The drawing under review shows one solid part. Ordinate dimensions are in mm from its lowest x, y, z. A direction names the side the tool comes from. Coordinates: 2 decimals unless noted, no trailing zeros. Write each loop counter-clockwise with the first axis right and the second up, starting at its lowest first coordinate (ties: lowest second). Pieces come first, ordered by that corner, then holes. Notation, with made-up numbers: (8.25, -16.75) -> (62.25, -16.75) arc R17 ccw to (62.25, -4.75) -> close; hole circle Ø10 at (76, 34). An arc over 180 degrees is marked (long way). One line per item, written item: value. Start each with the question number.
1) Add section D-D (y = 9). State the section outline as (x, z) points, and give its area (3 significant figures).
2) Mouldability with a two-part tool opening along X and no side actions: class the marked faces 1, 2 and 3 as released by +X, released by -X, zero draft, split by the parting line, or undercut.
3) For probe 1 along Y at (x, z) = (23, 1.9); probe 2 along X at (y, z) = (4, 13.5); probe 3 along Z at (x, y) = (23, 12.5), list the stretches that pass through material, from the lowest coordinate up. Write a range as from..to.
4) Add section A-A (z = 6.75). State the section outline as (x, y) points.
5) Add section B-B (x = 15). State the section outline as (y, z) points, and give its area (3 significant figures).
6) Add section C-C (y = 3). State the section outline as (x, z) points, and give its area (3 significant figures).
7) For pin 1 Ø2 at (x, y) = (30.5, 20) entering from +Z, flat-tipped, find the tip position at first contact; note if it passes through.
8) Machinability: for the marked faces 4 and 5, which of the approach directions +Z, -Z, +X, -X, +Y, -Y give a long, thin tool a straight path to every point of the face, cutting with its end or side? Answer none if there is none.
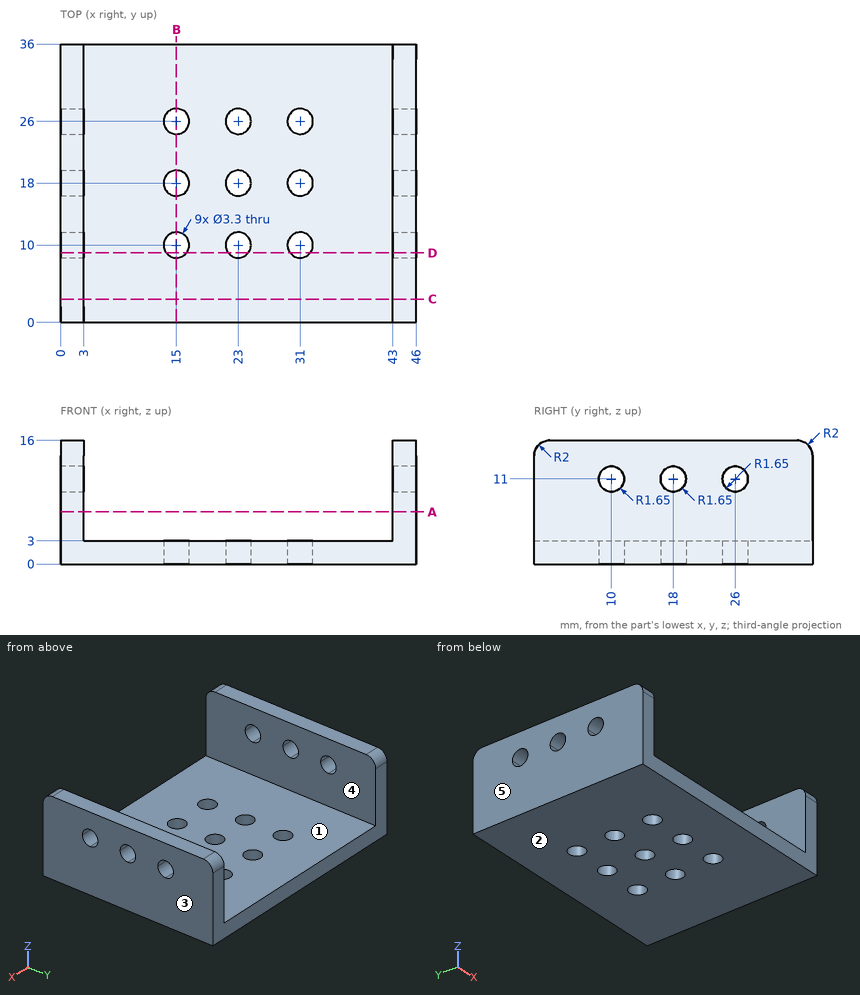
Numbers:
1. outline: (0, 0) -> (13.69, 0) -> (13.69, 3) -> (3, 3) -> (3, 9.69) -> (0, 9.69) -> close; (0, 12.31) -> (3, 12.31) -> (3, 16) -> (0, 16) -> close; (16.31, 0) -> (21.69, 0) -> (21.69, 3) -> (16.31, 3) -> close; (24.31, 0) -> (29.69, 0) -> (29.69, 3) -> (24.31, 3) -> close; (32.31, 0) -> (46, 0) -> (46, 9.69) -> (43, 9.69) -> (43, 3) -> (32.31, 3) -> close; (43, 12.31) -> (46, 12.31) -> (46, 16) -> (43, 16) -> close
1. area: 177 mm²
2. face 1: undercut
2. face 2: zero draft
2. face 3: released by +X
3. probe 1: 0..8.35, 11.65..16.35, 19.65..24.35, 27.65..36
3. probe 2: 0..3, 43..46
3. probe 3: 0..3
4. outline: (0, 0) -> (3, 0) -> (3, 36) -> (0, 36) -> close; (43, 0) -> (46, 0) -> (46, 36) -> (43, 36) -> close
5. outline: (0, 0) -> (8.35, 0) -> (8.35, 3) -> (0, 3) -> close; (11.65, 0) -> (16.35, 0) -> (16.35, 3) -> (11.65, 3) -> close; (19.65, 0) -> (24.35, 0) -> (24.35, 3) -> (19.65, 3) -> close; (27.65, 0) -> (36, 0) -> (36, 3) -> (27.65, 3) -> close
5. area: 78.3 mm²
6. outline: (0, 0) -> (46, 0) -> (46, 16) -> (43, 16) -> (43, 3) -> (3, 3) -> (3, 16) -> (0, 16) -> close
6. area: 216 mm²
7. pin 1: z = 3
8. face 4: +Z, +Y, -Y
8. face 5: +Z, -Z, -X, +Y, -Y
